Verification items for the finished model (mm, model axes). A direction names the side the tool comes from. Round coordinates to 2 decimals unless told otherwise and drop trailing zeros. Write each loop counter-clockwise with the first axis right and the second up, starting at its lowest first coordinate (ties: lowest second). Pieces come first, ordered by that corner, then holes.
from build123d import *

# Parameters (mm, degrees)
F1_DEPTH = 15.24
F2_R     = 4.445
F3_DEPTH = 50.8
F4_W     = 20.32
F4_H     = 3.302
F5_DEPTH = 15.24


with BuildPart() as f1:
    # F0 (on Top) → F1 (new body)
    with BuildSketch(Plane.XY):
        with BuildLine():
            ThreePointArc((31.75, 25.4), (28.030256, 34.380256), (19.05, 38.1))
            Line((19.05, 38.1), (-19.05, 38.1))
            ThreePointArc((-19.05, 38.1), (-28.030256, 34.380256), (-31.75, 25.4))
            Line((-31.75, 25.4), (-31.75, -25.4))
            ThreePointArc((-31.75, -25.4), (-28.030256, -34.380256), (-19.05, -38.1))
            Line((-19.05, -38.1), (19.05, -38.1))
            ThreePointArc((19.05, -38.1), (28.030256, -34.380256), (31.75, -25.4))
            Line((31.75, -25.4), (31.75, 25.4))
        make_face()
    extrude(amount=F1_DEPTH)

    # F2 (on face) → F3 (cut)
    with BuildSketch(Plane.XZ.offset(38.1)):
        with Locations((0, 7.62)):
            Circle(F2_R)
    extrude(amount=-F3_DEPTH, mode=Mode.SUBTRACT)

    # F4 (on face) → F5 (cut)
    with BuildSketch(Plane.XY.offset(15.24)):
        with Locations((0, 14.351)):
            Rectangle(F4_W, F4_H)
    extrude(amount=-F5_DEPTH, mode=Mode.SUBTRACT)


solid = f1.part
Q1. Sectioned sample at D-D (z = 11.25). Enter the section's corners in (x, y).
Recorded:
outline: (-31.75, -25.4) arc R12.7 ccw to (-19.05, -38.1) - (-2.57, -38.1) - (-2.57, 12.7) - (-10.16, 12.7) - (-10.16, 16) - (10.16, 16) - (10.16, 12.7) - (2.57, 12.7) - (2.57, -38.1) - (19.05, -38.1) arc R12.7 ccw to (31.75, -25.4) - (31.75, 25.4) arc R12.7 ccw to (19.05, 38.1) - (-19.05, 38.1) arc R12.7 ccw to (-31.75, 25.4) - close
Q2. Sectioned sample at C-C (z = 7.62). Enter the section's corners in (x, y) (3 decimals), plus the area to 3 significant figures.
Recorded:
outline: (-31.75, -25.4) arc R12.7 ccw to (-19.05, -38.1) - (-4.445, -38.1) - (-4.445, 12.7) - (-10.16, 12.7) - (-10.16, 16.002) - (10.16, 16.002) - (10.16, 12.7) - (4.445, 12.7) - (4.445, -38.1) - (19.05, -38.1) arc R12.7 ccw to (31.75, -25.4) - (31.75, 25.4) arc R12.7 ccw to (19.05, 38.1) - (-19.05, 38.1) arc R12.7 ccw to (-31.75, 25.4) - close
area: 4,180 mm2
Q3. Sectioned sample at B-B (x = 0). Enter the section's corners in (y, z) (3 decimals).
Recorded:
outline: (-38.1, 0) - (12.7, 0) - (12.7, 3.175) - (-38.1, 3.175) - close; (-38.1, 12.065) - (12.7, 12.065) - (12.7, 15.24) - (-38.1, 15.24) - close; (16.002, 0) - (38.1, 0) - (38.1, 15.24) - (16.002, 15.24) - close
Q4. Sectioned sample at A-A (y = 14). Enter the section's corners in (x, z), plus the area to 3 significant figures.
Recorded:
outline: (-31.75, 0) - (-10.16, 0) - (-10.16, 15.24) - (-31.75, 15.24) - close; (10.16, 0) - (31.75, 0) - (31.75, 15.24) - (10.16, 15.24) - close
area: 658 mm2
Q5. Material ranges on line 1 along Z through (x, y) = (0, -15) (3 decimals); line 2 along Y through (x, z) = (-5.5, 9.75); line 3 along Y through (x, z) = (1, 4.5), recorded low to high.
Recorded:
line 1: z = 0 to 3.175, 12.065 to 15.24
line 2: y = -38.1 to 12.7, 16 to 38.1
line 3: y = 16 to 38.1
Q6. Tool access check on faces 4 (the flat face through (0, 1, 15.24)), 5 (the cylindrical face through (-0.96, -13.06, 3.28)), 6 (the flat face through (10.16, 14, 8)). Record the directions out of +Z, -Z, +X, -X, +Y, -Y that give a thin tool (end or side, any length) a straight path to the whole face; none if there is none.
Recorded:
face 4: +Z, +X, -X, +Y, -Y
face 5: -Y
face 6: +Z, -Z
Q7. Release check for a two-part mould opening along Y. For faces 1 (the flat face through (-5, 12.7, 8)), 2 (the cylindrical face through (27.93, -34.48, 7.51)), 3 (the flat face through (0, 1, 0)) record: released by +Y, released by -Y, zero draft, split by the parting line, or undercut.
Recorded:
face 1: undercut
face 2: released by -Y
face 3: zero draft
